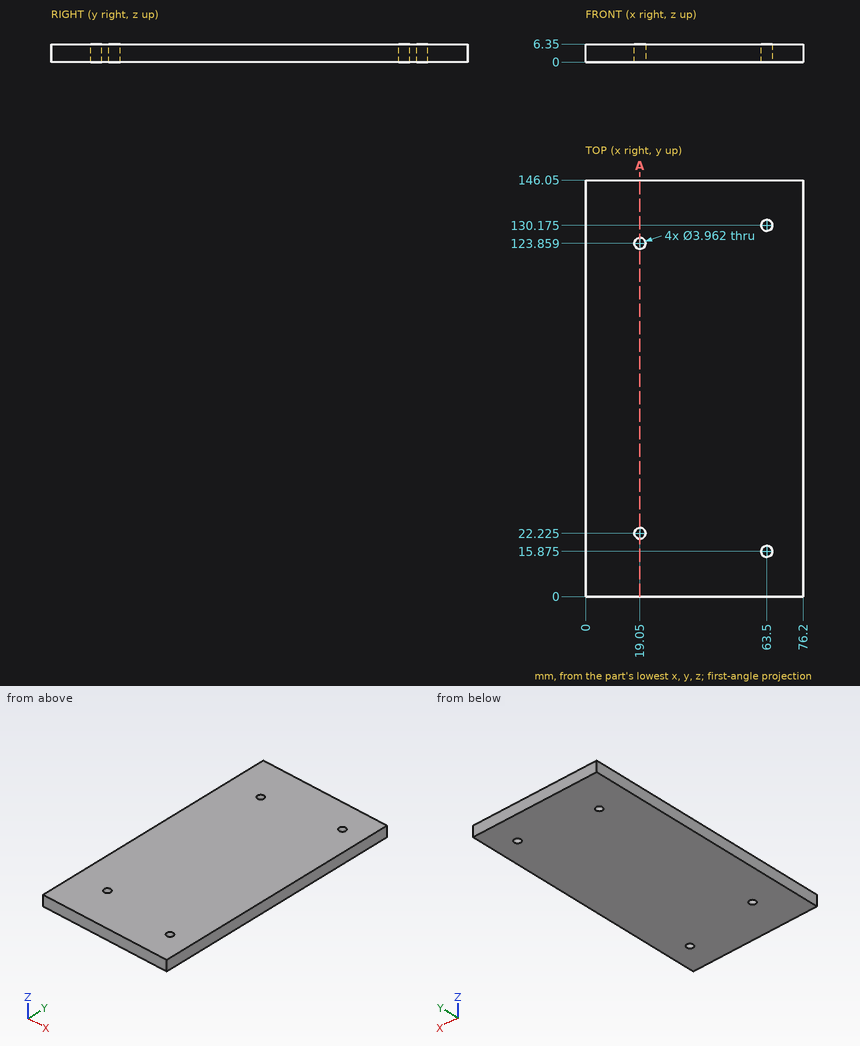
The figure shows three views and two pictorial views of one solid part (mm, origin at its lowest corner). Answer the questions. Round coordinates to 2 decimals unless told otherwise and drop trailing zeros. Order: outer loops, then holes, each group sorted by start corner. A loop starts at its lowest first (then second) coordinate and runs counter-clockwise, first axis right, second up. Notation, with made-up numbers: (38.25, 78) -> (47.25, 78) arc R11 cw to (47.25, 84) -> close; hole circle Ø5 at (61.25, 40). An arc over 180 degrees is marked (long way). One line per item, written item: value.
Item 1: Find section A-A, the plane x = 19.05. Give the vertices of the cut face in (y, z), then the cut area to 3 significant figures.
Taken from the geometry:
outline: (0, 0) -> (20.24, 0) -> (20.24, 6.35) -> (0, 6.35) -> close; (24.21, 0) -> (121.88, 0) -> (121.88, 6.35) -> (24.21, 6.35) -> close; (125.84, 0) -> (146.05, 0) -> (146.05, 6.35) -> (125.84, 6.35) -> close
area: 877 mm2
Item 2: Straight lines are drawn through the part: L1, parallel to Y at x = 19.05, z = 3; L2, parallel to Y at x = 63.5, z = 1.5; L3, parallel to X at y = 123.5, z = 2.75. For each, find the intervals that lie inside material, in ascending order.
Taken from the geometry:
L1: y = 0 to 20.24, 24.21 to 121.88, 125.84 to 146.05
L2: y = 0 to 13.89, 17.86 to 128.19, 132.16 to 146.05
L3: x = 0 to 17.1, 21 to 76.2
Item 3: Given P1, Ø3.5, axis at x = 63.5, y = 130.175, coming from the -Z side, flat-ended and moving along its own axis, determine where the tip first touches the part or whether it passes through.
Taken from the geometry:
P1: passes through
